from build123d import *

# Parameters (mm, degrees)
SKETCH_2_R      = 2.1
EXTRUDE_1_DEPTH = 400
FILLET_1_R      = 2
FILLET_2_R      = 0.2


with BuildPart() as part:
    # Эскиз2 → Бобышка-Вытянуть1 (new body)
    with BuildSketch(Plane(origin=(0, 0, 0), x_dir=(1, 0, 0), z_dir=(0, 1, 0))):
        Polygon((-10, -20), (-3.5, -20), (-3.5, -19), (-3, -19.005012563), (-3, -18.005012563), (-5.5, -18.005012563), (-5.5, -16.560660172), (-3, -14.060660172), (3, -14.060660172), (5.5, -16.560660172), (5.5, -18.005012563), (3, -18.005012563), (3, -19.005012563), (3.5, -19), (3.5, -20), (10, -20), (10, -13.5), (9, -13.5), (9.005012563, -13), (8.005012563, -13), (8.005012563, -15.5), (6.560660172, -15.5), (4.060660172, -13), (4.060660172, -7), (6.560660172, -4.5), (8.005012563, -4.5), (8.005012563, -7), (9.005012563, -7), (9, -6.5), (10, -6.5), (10, 6.5), (9, 6.5), (9.005012563, 7), (8.005012563, 7), (8.005012563, 4.5), (6.560660172, 4.5), (4.060660172, 7), (4.060660172, 13), (6.560660172, 15.5), (8.005012563, 15.5), (8.005012563, 13), (9.005012563, 13), (9, 13.5), (10, 13.5), (10, 20), (3.5, 20), (3.5, 19), (3, 19.005012563), (3, 18.005012563), (5.5, 18.005012563), (5.5, 16.560660172), (3, 14.060660172), (-3, 14.060660172), (-5.5, 16.560660172), (-5.5, 18.005012563), (-3, 18.005012563), (-3, 19.005012563), (-3.5, 19), (-3.5, 20), (-10, 20), (-10, 13.5), (-9, 13.5), (-9.005012563, 13), (-8.005012563, 13), (-8.005012563, 15.5), (-6.560660172, 15.5), (-4.060660172, 13), (-4.060660172, 7), (-6.560660172, 4.5), (-8.005012563, 4.5), (-8.005012563, 7), (-9.005012563, 7), (-9, 6.5), (-10, 6.5), (-10, -6.5), (-9, -6.5), (-9.005012563, -7), (-8.005012563, -7), (-8.005012563, -4.5), (-6.560660172, -4.5), (-4.060660172, -7), (-4.060660172, -13), (-6.560660172, -15.5), (-8.005012563, -15.5), (-8.005012563, -13), (-9.005012563, -13), (-9, -13.5), (-10, -13.5), align=None)
        with Locations(Location((0, 10, 0), (0, 0, 270))):
            Circle(SKETCH_2_R, mode=Mode.SUBTRACT)
        with Locations(Location((0, -10, 0), (0, 0, 90))):
            Circle(SKETCH_2_R, mode=Mode.SUBTRACT)
        Polygon((-2.764646715, 6.260660172), (2.764646715, 6.260660172), (5.920319141, 2.935275287), (8.005012563, 2.935275287), (8.005012563, -3.019020687), (5.920319141, -3.019020687), (2.678679656, -6.260660172), (-2.678679656, -6.260660172), (-5.920319141, -3.019020687), (-8.005012563, -3.019020687), (-8.005012563, 2.935275287), (-5.920319141, 2.935275287), align=None, mode=Mode.SUBTRACT)
    extrude(amount=EXTRUDE_1_DEPTH)

    # Скругление1
    fillet_1_edges = [part.edges().sort_by_distance(p)[0] for p in [
        (-10, 200, -20),
        (10, 200, -20),
        (10, 200, 20),
        (-10, 200, 20),
    ]]
    fillet(fillet_1_edges, radius=FILLET_1_R)

    # Скругление2
    fillet_2_edges = [part.edges().sort_by_distance(p)[0] for p in [
        (-9, 200, 13.5),
        (-9, 200, 6.5),
        (-9, 200, -6.5),
        (-9, 200, -13.5),
        (-3.5, 200, -19),
        (3.5, 200, -19),
        (9, 200, -13.5),
        (9, 200, -6.5),
        (9, 200, 6.5),
        (9, 200, 13.5),
        (3.5, 200, 19),
        (-3.5, 200, 19),
    ]]
    fillet(fillet_2_edges, radius=FILLET_2_R)


solid = part.part
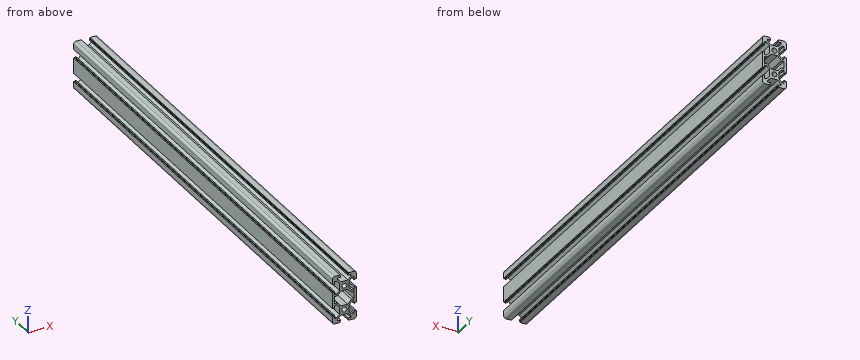
The listing builds one solid part. Answer for the finished solid, in the listing's coordinates (mm). Round coordinates to 2 decimals unless told otherwise and drop trailing zeros. Write item = value, one per line. Start each with the question number.
1) Section A-A, the plane y = 33 is taken. Count the separate pieces of the cut face and the enclosed holes in it, plus the area to 3 significant figures.
2) Straight lines are drawn through the part: L1, parallel to Z at x = -0.5, y = 356.5; L2, parallel to Z at x = 0.25, y = 291; L3, parallel to Z at x = -4.5, y = 143.5. For each, find the intervals that lie inside material, in ascending order.
3) Given pin 1 (0.8 mm diameter, centred on x = 8.5, y = 246.5, fed in from +Z); pin 2 (3 mm diameter, centred on y = 137.5, z = -10.5, fed in from -X); pin 3 (0.9 mm diameter, centred on x = 9.5, y = 108.5, fed in from +Z); pin 4 (2 mm diameter, centred on x = 5, z = -2, fed in from -Y), each flat-ended and moving along its own axis, determine where each tip first touches the part or whether it passes through.
Results list:
q1.separate_pieces = 1
q1.enclosed_holes = 3
q1.area = 316 mm^2
q2.L1 = -14.06 to -12.04, -7.96 to -6.26, 6.26 to 7.96, 12.04 to 14.06
q2.L2 = -14.06 to -12.09, -7.91 to -6.26, 6.26 to 7.91, 12.09 to 14.06
q2.L3 = -20 to -18.01, -15.56 to -13.44, -6.56 to -4.43, 4.44 to 6.56, 13.44 to 15.56, 18.01 to 20
q3.pin_1 = 20
q3.pin_2 = -4.06
q3.pin_3 = 19.7
q3.pin_4 = through
